Can you work these out from the model? Positions are in its coordinate system, mm. A direction names the side the tool comes from. Coordinates: 2 decimals unless noted, no trailing zeros. Order: outer loops, then holes, each group sorted by start corner. A loop starts at its lowest first (then second) coordinate and runs counter-clockwise, first axis right, second up. Notation, with made-up numbers: (23.5, 70) - (75.5, 70) arc R21 cw to (75.5, 101) - close; hole circle Ø11 at (80.25, 76). An arc over 180 degrees is marked (long way). Return JSON: item names as keys, results as strings. Group by question number.
1) Imagine slicing it at D-D (x = -110). Write out the boundary of the cut face in (y, z).
2) If we mould it in two halves opening along Y, with no side actions, what happens to faces 3 (the face through (0, -30, 27)), 4 (the face through (-82, -27.25, 28)), 5 (the face through (-44.65, -15, 28)), 6 (the face through (-61, 0, 27))? For each: pulls with the +Y half, pulls with the -Y half, needs draft (parallel to the pull), parting line crosses it, or undercut.
3) Imagine slicing it at A-A (z = 39.5). Write out the boundary of the cut face in (x, y).
4) Which directions (+Z, -Z, +X, -X, +Y, -Y) give clear straight access to the entire face, cutting with the end or side of a thin tool? Please do faces 1 (the face through (-82, -3, 28)), 2 (the face through (-61, -60.3, 27)).
5) If I drill on line 1 along Y through (x, z) = (-70.5, 31.5); line 2 along X through (y, z) = (-31.5, 36.5); line 3 along Y through (x, z) = (-6, 49), over which ranges is the centre line in solid material (lowest first)?
6) For pin 1 Ø1.5 at (x, y) = (-23.5, -6) entering from +Z, with a flat end and sliding along its axis, tell me the tip position at first contact or that it passes through.
7) Imagine slicing it at C-C (y = -14.5). Write out the boundary of the cut face in (x, z).
8) Imagine slicing it at B-B (x = -7.5). Write out the boundary of the cut face in (y, z), and give its area (3 significant figures).
```python
from build123d import *

# Parameters (mm, degrees)
F0_W     = 120.65
F0_H     = 60.3
F0_W_2   = 73
F0_H_2   = 27.05
F0_H_3   = 24.25
F0_W_3   = 38.65
F0_H_4   = 54.3
F1_DEPTH = 57
F2_W     = 120.65
F2_H     = 60.3
F2_W_2   = 73
F2_H_2   = 24.25
F2_H_3   = 27.05
F2_W_3   = 38.65
F2_H_4   = 54.3
F3_DEPTH = 3


with BuildPart() as f1:
    # F0 (on Top) → F1 (new body)
    with BuildSketch(Plane.XY):
        with Locations((-60.325, -30.15)):
            Rectangle(F0_W, F0_H)
        with Locations((-81.15, -43.775)):
            Rectangle(F0_W_2, F0_H_2, mode=Mode.SUBTRACT)
        with Locations((-81.15, -15.125)):
            Rectangle(F0_W_2, F0_H_3, mode=Mode.SUBTRACT)
        with Locations((-22.325, -30.15)):
            Rectangle(F0_W_3, F0_H_4, mode=Mode.SUBTRACT)
    extrude(amount=F1_DEPTH)

    # F2 (on face) → F3 (join)
    with BuildSketch(Plane(origin=(0, 0, 0), x_dir=(1, 0, 0), z_dir=(0, 0, -1))):
        with Locations((-60.325, 30.15)):
            Rectangle(F2_W, F2_H)
        with Locations((-81.15, 15.125)):
            Rectangle(F2_W_2, F2_H_2, mode=Mode.SUBTRACT)
        with Locations((-81.15, 43.775)):
            Rectangle(F2_W_2, F2_H_3, mode=Mode.SUBTRACT)
        with Locations((-22.325, 30.15)):
            Rectangle(F2_W_3, F2_H_4, mode=Mode.SUBTRACT)
        with Locations((-81.15, 43.775)):
            Rectangle(F2_W_2, F2_H_3)
        with Locations((-81.15, 15.125)):
            Rectangle(F2_W_2, F2_H_2)
        with Locations((-22.325, 30.15)):
            Rectangle(F2_W_3, F2_H_4)
    extrude(amount=F3_DEPTH)


solid = f1.part
```
Calculated:
{
 "1": {"outline": "(-60.3, -3) - (0, -3) - (0, 57) - (-3, 57) - (-3, 0) - (-27.25, 0) - (-27.25, 57) - (-30.25, 57) - (-30.25, 0) - (-57.3, 0) - (-57.3, 57) - (-60.3, 57) - close"},
 "2": {"face 3": "needs draft", "face 4": "undercut", "face 5": "undercut", "face 6": "pulls with the +Y half"},
 "3": {"outline": "(-120.65, -60.3) - (0, -60.3) - (0, 0) - (-120.65, 0) - close; hole (-117.65, -57.3) - (-44.65, -57.3) - (-44.65, -30.25) - (-117.65, -30.25) - close; hole (-117.65, -27.25) - (-44.65, -27.25) - (-44.65, -3) - (-117.65, -3) - close; hole (-41.65, -57.3) - (-3, -57.3) - (-3, -3) - (-41.65, -3) - close"},
 "4": {"face 1": "+Z", "face 2": "+Z, -Z, +X, -X, -Y"},
 "5": {"line 1": "-60.3 to -57.3, -30.25 to -27.25, -3 to 0", "line 2": "-120.65 to -117.65, -44.65 to -41.65, -3 to 0", "line 3": "-60.3 to -57.3, -3 to 0"},
 "6": {"pin 1": "z = 0"},
 "7": {"outline": "(-120.65, -3) - (0, -3) - (0, 57) - (-3, 57) - (-3, 0) - (-41.65, 0) - (-41.65, 57) - (-44.65, 57) - (-44.65, 0) - (-117.65, 0) - (-117.65, 57) - (-120.65, 57) - close"},
 "8": {"outline": "(-60.3, -3) - (0, -3) - (0, 57) - (-3, 57) - (-3, 0) - (-57.3, 0) - (-57.3, 57) - (-60.3, 57) - close", "area": "523 mm2"}
}
